Part model, mm, in its own coordinate system. A direction names the side the tool comes from. Round coordinates to 2 decimals unless told otherwise and drop trailing zeros. Order: outer loops, then holes, each group sorted by start corner. A loop starts at its lowest first (then second) coordinate and runs counter-clockwise, first axis right, second up. Notation, with made-up numbers: (18, 31.5) - (53, 31.5) arc R37 cw to (53, 67.5) - close; hole circle Ø5 at (85, 32). An arc over 180 degrees is marked (long way). Answer as a JSON object with one key per item and string values.
```python
from build123d import *

# Parameters (mm, degrees)
SKETCH1_R           = 2.8
SKETCH1_R_2         = 1.5
BOSS_EXTRUDE1_DEPTH = 5
SKETCH2_R           = 2.8
BOSS_EXTRUDE2_DEPTH = 30
SKETCH3_R           = 2.8
SKETCH3_R_2         = 1.5
BOSS_EXTRUDE3_DEPTH = 5


with BuildPart() as part:
    # Sketch1 → Boss-Extrude1 (new body)
    with BuildSketch(Plane.XY):
        Circle(SKETCH1_R)
        Circle(SKETCH1_R_2, mode=Mode.SUBTRACT)
    extrude(amount=BOSS_EXTRUDE1_DEPTH)

    # Sketch2 → Boss-Extrude2 (add)
    with BuildSketch(Plane.XY.offset(5)):
        Circle(SKETCH2_R)
    extrude(amount=BOSS_EXTRUDE2_DEPTH)

    # Sketch3 → Boss-Extrude3 (add)
    with BuildSketch(Plane.XY.offset(35)):
        Circle(SKETCH3_R)
        Circle(SKETCH3_R_2, mode=Mode.SUBTRACT)
    extrude(amount=BOSS_EXTRUDE3_DEPTH)


solid = part.part
```
Item 1: Probe L1, parallel to Y at x = 0, z = 3.3; L2, parallel to Z at x = -0.7, y = 0.65; L3, parallel to X at y = -0.95, z = 3. List the from-to ranges inside material, lowest first. Write a range as from..to.
Taken from the geometry:
{"L1": "-2.8..-1.5, 1.5..2.8", "L2": "5..35", "L3": "-2.63..-1.16, 1.16..2.63"}
Item 2: Cut at D-D (z = 30). Write the cut outline in (x, y), plus the area to 3 significant figures.
Taken from the geometry:
{"outline": "circle Ø5.6 at (0, 0)", "area": "24.6 mm2"}
Item 3: Cut at A-A (x = 0). Write the cut outline in (y, z), plus the area to 3 significant figures.
Taken from the geometry:
{"outline": "(-2.8, 0) - (-1.5, 0) - (-1.5, 5) - (1.5, 5) - (1.5, 0) - (2.8, 0) - (2.8, 40) - (1.5, 40) - (1.5, 35) - (-1.5, 35) - (-1.5, 40) - (-2.8, 40) - close", "area": "194 mm2"}
Item 4: Tool access for faces 1 (the cylindrical face through (-1.5, 0.07, 37.47)), 2 (the flat face through (1.2, -1.2, 40)): list every direction of +Z, -Z, +X, -X, +Y, -Y with a clear straight run to the whole face (end or side of a thin tool).
Taken from the geometry:
{"face 1": "+Z", "face 2": "+Z, +X, -X, +Y, -Y"}
Item 5: Drop flat-ended pins along their axis: P1, Ø2.5, axis at x = 0, y = 0, coming from the -Z side; P2, Ø2.5, axis at x = 0, y = 0, coming from the +Z side. Give the stop position or say it passes through.
Taken from the geometry:
{"P1": "z = 5", "P2": "z = 35"}
Item 6: Cut at B-B (z = 35.5). Write the cut outline in (x, y), plus the area to 3 significant figures.
Taken from the geometry:
{"outline": "circle Ø5.6 at (0, 0); hole circle Ø3 at (0, 0)", "area": "17.6 mm2"}
Item 7: Cut at C-C (y = 1.1). Write the cut outline in (x, z), plus the area to 3 significant figures.
Taken from the geometry:
{"outline": "(-2.57, 0) - (-1.02, 0) - (-1.02, 5) - (1.02, 5) - (1.02, 0) - (2.57, 0) - (2.57, 40) - (1.02, 40) - (1.02, 35) - (-1.02, 35) - (-1.02, 40) - (-2.57, 40) - close", "area": "186 mm2"}
Item 8: Two-plate mould, pull along X, no slides. Class faces 3 (the flat face through (1.2, -1.2, 0)), 4 (the cylindrical face through (-1.5, 0.07, 2.46)), 5 (the cylindrical face through (-2.8, 0.1, 19.7)), 6 (the flat face through (0, 0, 5)): pulls with the +X half, pulls with the -X half, needs draft (parallel to the pull), parting line crosses it, or undercut.
Taken from the geometry:
{"face 3": "needs draft", "face 4": "undercut", "face 5": "parting line crosses it", "face 6": "undercut"}
